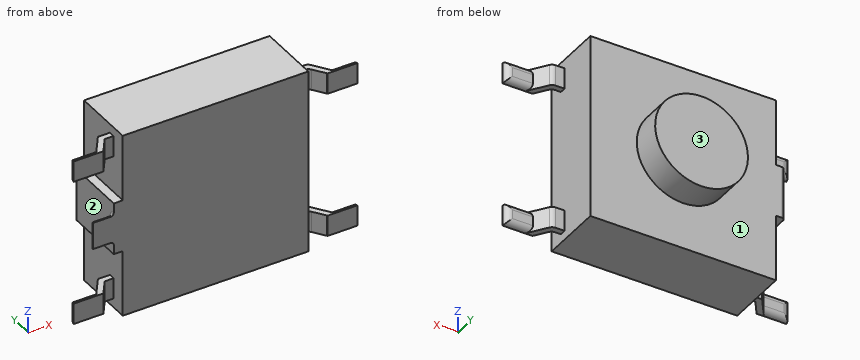
from build123d import *

# Parameters (mm, degrees)
ESQUISSE1_W         = 6.2
ESQUISSE1_H         = 6.2
BOSS_EXTRU_1_DEPTH  = 2.1
ESQUISSE2_R         = 1.55
BOSS_EXTRU_2_DEPTH  = 1
ESQUISSE3_W         = 1.75
ESQUISSE3_H         = 2.1
BOSS_EXTRU_3_DEPTH  = 0.3
ESQUISSE4_W         = 0.9
ESQUISSE4_H         = 0.1
BOSS_EXTRU_4_DEPTH  = 0.7
CONG_1_R            = 0.1
ESQUISSE5_W         = 0.7
ESQUISSE5_H         = 0.2
BOSS_EXTRU_5_DEPTH  = 0.4
ESQUISSE7_W         = 0.7
ESQUISSE7_H         = 0.2
BOSS_EXTRU_6_DEPTH  = 0.7
CONG_2_R            = 0.2
ESQUISSE9_W         = 1
ESQUISSE9_H         = 0.7
BOSS_EXTRU_7_DEPTH  = 0.2
CONG_3_R            = 0.2
CONG_4_R            = 0.2
ESQUISSE10_W        = 0.7
ESQUISSE10_H        = 0.2
BOSS_EXTRU_10_DEPTH = 0.4
ESQUISSE14_W        = 0.7
ESQUISSE14_H        = 0.2
BOSS_EXTRU_11_DEPTH = 0.7
ESQUISSE16_W        = 1
ESQUISSE16_H        = 0.7
BOSS_EXTRU_12_DEPTH = 0.2
CONG_5_R            = 0.2


with BuildPart() as part:
    # Esquisse1 → Boss.-Extru.1 (new body)
    with BuildSketch(Plane(origin=(0, 0, 0), x_dir=(1, 0, 0), z_dir=(0, 1, 0))):
        with Locations((3.1, 3.1)):
            Rectangle(ESQUISSE1_W, ESQUISSE1_H)
    extrude(amount=BOSS_EXTRU_1_DEPTH)

    # Esquisse2 → Boss.-Extru.2 (add)
    with BuildSketch(Plane(origin=(0, 2.1, 0), x_dir=(1, 0, 0), z_dir=(0, 1, 0))):
        with Locations(Location((3.1, 3.1, 0), (0, 0, 90))):
            Circle(ESQUISSE2_R)
    extrude(amount=BOSS_EXTRU_2_DEPTH)

    # Esquisse3 → Boss.-Extru.3 (add)
    with BuildSketch(Plane.ZY):
        with Locations((-3.1, 1.05)):
            Rectangle(ESQUISSE3_W, ESQUISSE3_H)
    extrude(amount=BOSS_EXTRU_3_DEPTH)

    # Esquisse4 → Boss.-Extru.4 (add)
    with BuildSketch(Plane.ZY.offset(0.3)):
        with Locations((-3.1, 0.05)):
            Rectangle(ESQUISSE4_W, ESQUISSE4_H)
    extrude(amount=BOSS_EXTRU_4_DEPTH)

    # Congé1
    cong_1_edges = [part.edges().sort_by_distance(p)[0] for p in [
        (-0.65, 0.1, -3.55),
        (-0.65, 0.1, -2.65),
        (-1, 0.1, -3.1),
        (-0.3, 2.1, -3.1),
    ]]
    fillet(cong_1_edges, radius=CONG_1_R - 0.0001)  # a hair under: the kernel refuses the full size
    cong_1_2_edges = [part.edges().sort_by_distance(p)[0] for p in [
        (-0.3, 0.1, -3.1),
        (-0.3, 0.070739967, -3.520739967),
        (-0.3, 0.070739967, -2.679260033),
    ]]
    fillet(cong_1_2_edges, radius=CONG_1_R)

    # Esquisse5 → Boss.-Extru.5 (add)
    with BuildSketch(Plane(origin=(6.2, 0, 0), x_dir=(0, 0, -1), z_dir=(1, 0, 0))):
        with Locations((0.65, 0.6)):
            Rectangle(ESQUISSE5_W, ESQUISSE5_H)
        with Locations((5.55, 0.6)):
            Rectangle(ESQUISSE5_W, ESQUISSE5_H)
    extrude(amount=BOSS_EXTRU_5_DEPTH)

    # Esquisse7 → Boss.-Extru.6 (add)
    with BuildSketch(Plane(origin=(1.84244111, -2.631278598, 0), x_dir=(0, 0, -1), z_dir=(-0.5735764363510502, 0.8191520442889889, 0))):
        with Locations((5.55, -5.707906998)):
            Rectangle(ESQUISSE7_W, ESQUISSE7_H)
        with Locations((0.65, -5.707906998)):
            Rectangle(ESQUISSE7_W, ESQUISSE7_H)
    extrude(amount=-BOSS_EXTRU_6_DEPTH)

    # Congé2
    cong_2_edges = [part.edges().sort_by_distance(p)[0] for p in [
        (6.49588659, 0.5, -5.55),
        (6.49588659, 0.5, -0.65),
        (6.6, 0.7, -0.65),
        (6.6, 0.7, -5.55),
    ]]
    fillet(cong_2_edges, radius=CONG_2_R)

    # Esquisse9 → Boss.-Extru.7 (add)
    with BuildSketch(Plane(origin=(0, 0, 0), x_dir=(1, 0, 0), z_dir=(0, 1, 0))):
        with Locations((7.337673097, 0.65)):
            Rectangle(ESQUISSE9_W, ESQUISSE9_H)
        with Locations((7.337673097, 5.55)):
            Rectangle(ESQUISSE9_W, ESQUISSE9_H)
    extrude(amount=BOSS_EXTRU_7_DEPTH)

    # Congé3
    cong_3_edges = [part.edges().sort_by_distance(p)[0] for p in [
        (7.837673097, 0.2, -0.65),
        (7.393888433, 0.2, -1),
        (7.393888433, 0.2, -0.3),
    ]]
    fillet(cong_3_edges, radius=CONG_3_R - 0.0001)  # a hair under: the kernel refuses the full size

    # Congé4
    cong_4_edges = [part.edges().sort_by_distance(p)[0] for p in [
        (7.393888433, 0.2, -5.9),
        (7.837673097, 0.2, -5.55),
        (7.393888433, 0.2, -5.2),
    ]]
    fillet(cong_4_edges, radius=CONG_4_R - 0.0001)  # a hair under: the kernel refuses the full size

    # Esquisse10 → Boss.-Extru.10 (add)
    with BuildSketch(Plane.ZY):
        with Locations((-5.55, 0.6)):
            Rectangle(ESQUISSE10_W, ESQUISSE10_H)
        with Locations((-0.65, 0.6)):
            Rectangle(ESQUISSE10_W, ESQUISSE10_H)
    extrude(amount=BOSS_EXTRU_10_DEPTH)

    # Esquisse14 → Boss.-Extru.11 (add)
    with BuildSketch(Plane(origin=(0.197296446, 0.281768526, 0), x_dir=(0, 0, -1), z_dir=(-0.5735764363510527, -0.8191520442889871, 0))):
        with Locations((0.65, -0.629164323)):
            Rectangle(ESQUISSE14_W, ESQUISSE14_H)
        with Locations((5.55, -0.629164323)):
            Rectangle(ESQUISSE14_W, ESQUISSE14_H)
    extrude(amount=BOSS_EXTRU_11_DEPTH)

    # Esquisse16 → Boss.-Extru.12 (add)
    with BuildSketch(Plane(origin=(0, 0, 0), x_dir=(1, 0, 0), z_dir=(0, 1, 0))):
        with Locations((-1.137673097, 0.65)):
            Rectangle(ESQUISSE16_W, ESQUISSE16_H)
        with Locations((-1.137673097, 5.55)):
            Rectangle(ESQUISSE16_W, ESQUISSE16_H)
    extrude(amount=BOSS_EXTRU_12_DEPTH)

    # Congé5
    cong_5_edges = [part.edges().sort_by_distance(p)[0] for p in [
        (-1.193888433, 0.2, -5.9),
        (-1.637673097, 0.2, -5.55),
        (-1.193888433, 0.2, -5.2),
        (-1.193888433, 0.2, -1),
        (-1.637673097, 0.2, -0.65),
        (-1.193888433, 0.2, -0.3),
    ]]
    fillet(cong_5_edges, radius=CONG_5_R - 0.0001)  # a hair under: the kernel refuses the full size


solid = part.part
CAD build for the part. Positions are in the model's coordinates, mm. Face numbers are marked on the shaded views. A direction names the side the tool comes from. Round coordinates to 2 decimals unless told otherwise and drop trailing zeros. Write each loop counter-clockwise with the first axis right and the second up, starting at its lowest first coordinate (ties: lowest second). Pieces come first, ordered by that corner, then holes. Notation, with made-up numbers: M -35,-21 L 2,-21 A27 ccw 2,1 Z; hole C 4,28.25 d6. An arc over 180 degrees is marked long. Use a Markdown table: item, result. Add a question column.
1. Slice it at A-A on y = 1. Give the cut face in (x, z) (3 decimals), then the cut area to 3 significant figures.
2. Slice it at B-B on x = 3.1. Give the cut face in (y, z).
3. Flat gauge pins, fed straight in: P1, Ø1, axis at y = 1.5, z = -0.5, coming from the -X side; P2, Ø0.6, axis at x = -0.5, y = 0, coming from the -Z side; P3, Ø1.5, axis at x = -0.5, y = 1.5, coming from the -Z side; P4, Ø1.5, axis at x = 1, z = -2, coming from the +Y side. Where does each tip first touch, or does it go through?
4. Drill centre lines: probe 1 along Y at (x, z) = (5.25, -5); probe 2 along X at (y, z) = (0.2, -1.5); probe 3 along X at (y, z) = (1.5, -3.5). Where is each one in solid material? Low to high.
5. 3-axis set-ups, long thin cutter, end or side, ignore diameter. For the marked faces 1, 2 and 3: which of +Z, -Z, +X, -X, +Y, -Y reach the whole face in a straight line?
Reply:
| question | item | result |
|---|---|---|
| 1 | outline | M -0.3,-3.975 L 0,-3.975 L 0,-6.2 L 6.2,-6.2 L 6.2,0 L 0,0 L 0,-2.225 L -0.3,-2.225 Z |
| 1 | area | 39.0 mm^2 |
| 2 | outline | M 0,-6.2 L 2.1,-6.2 L 2.1,-4.65 L 3.1,-4.65 L 3.1,-1.55 L 2.1,-1.55 L 2.1,0 L 0,0 Z |
| 3 | P1 | stops at x = 0 |
| 3 | P2 | stops at z = -5.9 |
| 3 | P3 | stops at z = -6.2 |
| 3 | P4 | stops at y = 2.1 |
| 4 | probe 1 | y = 0 to 2.1 |
| 4 | probe 2 | x = 0 to 6.2 |
| 4 | probe 3 | x = -0.3 to 6.2 |
| 5 | face 1 | +Y |
| 5 | face 2 | -X, +Y |
| 5 | face 3 | +Z, -Z, +X, -X, +Y |
